```python
from build123d import *

# Parameters (mm, degrees)
BOSS_EXTRUDE3_DEPTH = 34
CUT_EXTRUDE4_DEPTH  = 17


with BuildPart() as part:
    # Sketch12 → Boss-Extrude3 (new body)
    with BuildSketch(Plane.XY):
        with BuildLine():
            Line((30.5, -9.25), (-30.5, -9.25))
            ThreePointArc((-30.5, -9.25), (-34.035533906, -7.785533906), (-35.5, -4.25))
            Line((-35.5, -4.25), (-35.5, 4.25))
            ThreePointArc((-35.5, 4.25), (-34.035533906, 7.785533906), (-30.5, 9.25))
            Line((-30.5, 9.25), (30.5, 9.25))
            ThreePointArc((30.5, 9.25), (34.035533906, 7.785533906), (35.5, 4.25))
            Line((35.5, 4.25), (35.5, -4.25))
            ThreePointArc((35.5, -4.25), (34.035533906, -7.785533906), (30.5, -9.25))
        make_face()
        with BuildLine():
            Line((29.5, -8.25), (-29.5, -8.25))
            ThreePointArc((-29.5, -8.25), (-33.035533906, -6.785533906), (-34.5, -3.25))
            Line((-34.5, -3.25), (-34.5, 3.25))
            ThreePointArc((-34.5, 3.25), (-33.035533906, 6.785533906), (-29.5, 8.25))
            Line((-29.5, 8.25), (29.5, 8.25))
            ThreePointArc((29.5, 8.25), (33.035533906, 6.785533906), (34.5, 3.25))
            Line((34.5, 3.25), (34.5, -3.25))
            ThreePointArc((34.5, -3.25), (33.035533906, -6.785533906), (29.5, -8.25))
        make_face(mode=Mode.SUBTRACT)
    extrude(amount=BOSS_EXTRUDE3_DEPTH)

    # Sketch14 → Cut-Extrude4 (cut, symmetric)
    with BuildSketch(Plane(origin=(0, 0, 0), x_dir=(1, 0, 0), z_dir=(0, 1, 0))):
        with BuildLine():
            ThreePointArc((-34.5, 0), (-35.207106781, -0.292893219), (-35.5, -1))
            Line((-35.5, -1), (-35.5, 0))
            Line((-35.5, 0), (-34.5, 0))
        make_face()
        with BuildLine():
            Line((34.5, 0), (35.5, 0))
            Line((35.5, 0), (35.5, -1))
            ThreePointArc((35.5, -1), (35.207106781, -0.292893219), (34.5, 0))
        make_face()
        with BuildLine():
            ThreePointArc((34.5, -34), (35.207106781, -33.707106781), (35.5, -33))
            Line((35.5, -33), (35.5, -34))
            Line((35.5, -34), (34.5, -34))
        make_face()
        with BuildLine():
            ThreePointArc((-35.5, -33), (-35.207106781, -33.707106781), (-34.5, -34))
            Line((-34.5, -34), (-35.5, -34))
            Line((-35.5, -34), (-35.5, -33))
        make_face()
    extrude(amount=CUT_EXTRUDE4_DEPTH, both=True, mode=Mode.SUBTRACT)


solid = part.part
```
The listing builds one solid part. Answer for the finished solid, in the listing's coordinates (mm). A direction names the side the tool comes from. Give positions to 0.01 mm unless a question says otherwise; leave off trailing zeros. Order: outer loops, then holes, each group sorted by start corner. A loop starts at its lowest first (then second) coordinate and runs counter-clockwise, first axis right, second up. Notation, with made-up numbers: M -1.75,69 L 29.25,69 A20 cw 29.25,80 Z; hole C -5,77.5 d9. An arc over 180 degrees is marked long. Put each result on its own line as item: value. Start each with the question number.
Item 1: Which of the six approach directions +Z, -Z, +X, -X, +Y, -Y give full straight-line access (tool end or side, diameter ignored) to faces 1 (the face through (0, 9, 0)), 2 (the face through (0, -8.25, 17))?
Item 2: The part is cut by section C-C, the plane z = 6.5. Determine the outline of the cut face in (x, y), and give its area (3 significant figures).
Item 3: The part is cut by section B-B, the plane y = 6.25. Determine the outline of the cut face in (x, z).
Item 4: The part is cut by section D-D, the plane y = -5. Determine the outline of the cut face in (x, z), and give its area (3 significant figures).
Item 5: A flat-ended cylindrical pin translates along its axis: P1, Ø5, axis at y = 7, z = 29, coming from the +X side. Find the tip coordinate at first contact, or state that the pin passes through.
Item 6: Find the intervals of material crossed by line 1 along X through (y, z) = (-3, 17); line 2 along Y through (x, z) = (-22, 4), in increasing order.
Item 7: The part is cut by section A-A, the plane x = -6. Determine the outline of the cut face in (y, z), and give its area (3 significant figures).
Answer key:
1. face 1: -Z, +X, -X, +Y, -Y
1. face 2: +Z, -Z
2. outline: M -35.5,-4.25 A5 ccw -30.5,-9.25 L 30.5,-9.25 A5 ccw 35.5,-4.25 L 35.5,4.25 A5 ccw 30.5,9.25 L -30.5,9.25 A5 ccw -35.5,4.25 Z; hole M -34.5,-3.25 A5 ccw -29.5,-8.25 L 29.5,-8.25 A5 ccw 34.5,-3.25 L 34.5,3.25 A5 ccw 29.5,8.25 L -29.5,8.25 A5 ccw -34.5,3.25 Z
2. area: 175 mm²
3. outline: M -35.08,0.19 A1 ccw -34.5,0 L -33.5,0 L -33.5,34 L -34.5,34 A1 ccw -35.08,33.81 Z; M 33.5,0 L 34.5,0 A1 ccw 35.08,0.19 L 35.08,33.81 A1 ccw 34.5,34 L 33.5,34 Z
4. outline: M -35.44,0.67 A1 ccw -34.5,0 L -34.18,0 L -34.18,34 L -34.5,34 A1 ccw -35.44,33.33 Z; M 34.18,0 L 34.5,0 A1 ccw 35.44,0.67 L 35.44,33.33 A1 ccw 34.5,34 L 34.18,34 Z
4. area: 85.0 mm²
5. P1: stops at x = 35.49
6. line 1: x = -35.5 to -34.5, 34.5 to 35.5
6. line 2: y = -9.25 to -8.25, 8.25 to 9.25
7. outline: M -9.25,0 L -8.25,0 L -8.25,34 L -9.25,34 Z; M 8.25,0 L 9.25,0 L 9.25,34 L 8.25,34 Z
7. area: 68.0 mm²
